Here's how the part is built. I have some questions about the finished solid (model axes, mm). Coordinates: 2 decimals unless noted, no trailing zeros. Answer in a Markdown table with one row per item. Add a question column.
from build123d import *

# Parameters (mm, degrees)
ESQUISSE1_W             = 20
ESQUISSE1_H             = 530
BOSS_EXTRU_1_DEPTH      = 11
ENL_V_MAT_EXTRU_1_DEPTH = 531.208449574
ENL_V_MAT_EXTRU_2_DEPTH = 531.208449574
ENL_V_MAT_EXTRU_3_DEPTH = 531.208449574
ENL_V_MAT_EXTRU_4_DEPTH = 531.208449574
PER_AGE1_D              = 4.917
PER_AGE2_D              = 4.917
CHANFREIN1_SIZE         = 0.5415
CHANFREIN2_SIZE         = 0.3


with BuildPart() as part:
    # Esquisse1 → Boss.-Extru.1 (new body)
    with BuildSketch(Plane.XZ):
        with Locations((0, -15)):
            Rectangle(ESQUISSE1_W, ESQUISSE1_H)
    extrude(amount=-BOSS_EXTRU_1_DEPTH)

    # Esquisse2 → Enlèv. mat.-Extru.1 (cut, through all)
    with BuildSketch(Plane(origin=(0, 0, -280), x_dir=(-1, 0, 0), z_dir=(0, 0, -1))):
        with BuildLine():
            Line((10, 7.9), (10, 10.22385))
            Line((10, 10.22385), (9.440021531, 9.900556887))
            ThreePointArc((9.440021531, 9.900556887), (9.015681976, 9.557293765), (8.71772889, 9.1))
            Line((8.71772889, 9.1), (7.5, 9.1))
            Line((7.5, 9.1), (7.5, 7.9))
            Line((7.5, 7.9), (10, 7.9))
        make_face()
    extrude(amount=-ENL_V_MAT_EXTRU_1_DEPTH, mode=Mode.SUBTRACT)

    # Esquisse3 → Enlèv. mat.-Extru.2 (cut, through all)
    with BuildSketch(Plane(origin=(0, 0, -280), x_dir=(-1, 0, 0), z_dir=(0, 0, -1))):
        with BuildLine():
            Line((9.440021531, 7.099443113), (10, 6.77615))
            Line((10, 6.77615), (10, 7.9))
            Line((10, 7.9), (8.71772889, 7.9))
            ThreePointArc((8.71772889, 7.9), (9.015681976, 7.442706235), (9.440021531, 7.099443113))
        make_face()
    extrude(amount=-ENL_V_MAT_EXTRU_2_DEPTH, mode=Mode.SUBTRACT)

    # Esquisse4 → Enlèv. mat.-Extru.3 (cut, through all)
    with BuildSketch(Plane(origin=(0, 0, -280), x_dir=(-1, 0, 0), z_dir=(0, 0, -1))):
        with BuildLine():
            Line((-10, 9.1), (-10, 6.77615))
            Line((-10, 6.77615), (-9.440021531, 7.099443113))
            ThreePointArc((-9.440021531, 7.099443113), (-9.015681976, 7.442706235), (-8.71772889, 7.9))
            Line((-8.71772889, 7.9), (-7.5, 7.9))
            Line((-7.5, 7.9), (-7.5, 9.1))
            Line((-7.5, 9.1), (-10, 9.1))
        make_face()
    extrude(amount=-ENL_V_MAT_EXTRU_3_DEPTH, mode=Mode.SUBTRACT)

    # Esquisse5 → Enlèv. mat.-Extru.4 (cut, through all)
    with BuildSketch(Plane(origin=(0, 0, -280), x_dir=(-1, 0, 0), z_dir=(0, 0, -1))):
        with BuildLine():
            Line((-9.440021531, 9.900556887), (-10, 10.22385))
            Line((-10, 10.22385), (-10, 9.1))
            Line((-10, 9.1), (-8.71772889, 9.1))
            ThreePointArc((-8.71772889, 9.1), (-9.015681976, 9.557293765), (-9.440021531, 9.900556887))
        make_face()
    extrude(amount=-ENL_V_MAT_EXTRU_4_DEPTH, mode=Mode.SUBTRACT)

    # Perçage1 (through all)
    with Locations(Plane(origin=(0, 11, 0), x_dir=(1, 0, 0), z_dir=(0, 1, 0))):
        with Locations((0, -180), (0, -120), (0, 60), (0, 180)):
            Hole(PER_AGE1_D / 2)

    # Perçage2 (through all)
    with Locations(Plane(origin=(0, 0, 0), x_dir=(-1, 0, 0), z_dir=(0, -1, 0))):
        with Locations((0, -240), (0, -60), (0, 0), (0, 120), (0, 240)):
            Hole(PER_AGE2_D / 2)

    # Chanfrein1
    chanfrein1_edges = [part.edges().sort_by_distance(p)[0] for p in [
        (2.4585, 11, 180),
        (2.4585, 0, 180),
        (-2.4585, 0, -240),
        (-2.4585, 11, -240),
        (-2.4585, 0, -120),
        (-2.4585, 11, -120),
        (-2.4585, 0, 0),
        (-2.4585, 11, 0),
        (-2.4585, 0, 60),
        (-2.4585, 11, 60),
        (-2.4585, 0, 240),
        (-2.4585, 11, 240),
        (10, 0, -15),
        (-10, 0, -15),
        (2.4585, 11, -180),
        (2.4585, 0, -180),
        (2.4585, 11, -60),
        (2.4585, 0, -60),
        (2.4585, 11, 120),
        (2.4585, 0, 120),
    ]]
    chamfer(chanfrein1_edges, length=CHANFREIN1_SIZE)

    # Chanfrein2
    chanfrein2_edges = [part.edges().sort_by_distance(p)[0] for p in [
        (10, 11, -15),
        (-10, 11, -15),
    ]]
    chamfer(chanfrein2_edges, length=CHANFREIN2_SIZE)


solid = part.part
Q1. I'm going to push flat-ended pins straight in: P1, Ø5.5, axis at x = 0, z = -240, coming from the +Y side; P2, Ø8, axis at x = 0, z = -60, coming from the +Y side; P3, Ø5.5, axis at x = 0, z = 0, coming from the -Y side; P4, Ø2, axis at y = 9, z = -187, coming from the +X side. Where does each tip first touch, or does it pass through?
Q2. Imagine slicing it at A-A on y = 5. State how many separate pieces and enclosed holes the cut face has, plus the area to 3 significant figures.
Q3. I need wall thicknesses on line 1 (Y direction, x = 9, z = 109); line 2 (X direction, y = 8.25, z = -60); line 3 (X direction, y = 5.5, z = -120). Which ranges of each line are inside material? Lowest first, please. Write a range as [from, to].
Result sheet:
| question | item | result |
|---|---|---|
| 1 | P1 | stops at y = 10.75 |
| 1 | P2 | stops at y = 11 |
| 1 | P3 | stops at y = 0.25 |
| 1 | P4 | stops at x = 9.61 |
| 2 | separate pieces | 1 |
| 2 | enclosed holes | 9 |
| 2 | area | 10,400 mm^2 |
| 3 | line 1 | y = [0, 7.46], [9.54, 11] |
| 3 | line 2 | x = [-7.5, -2.46], [2.46, 7.5] |
| 3 | line 3 | x = [-10, -2.46], [2.46, 10] |
